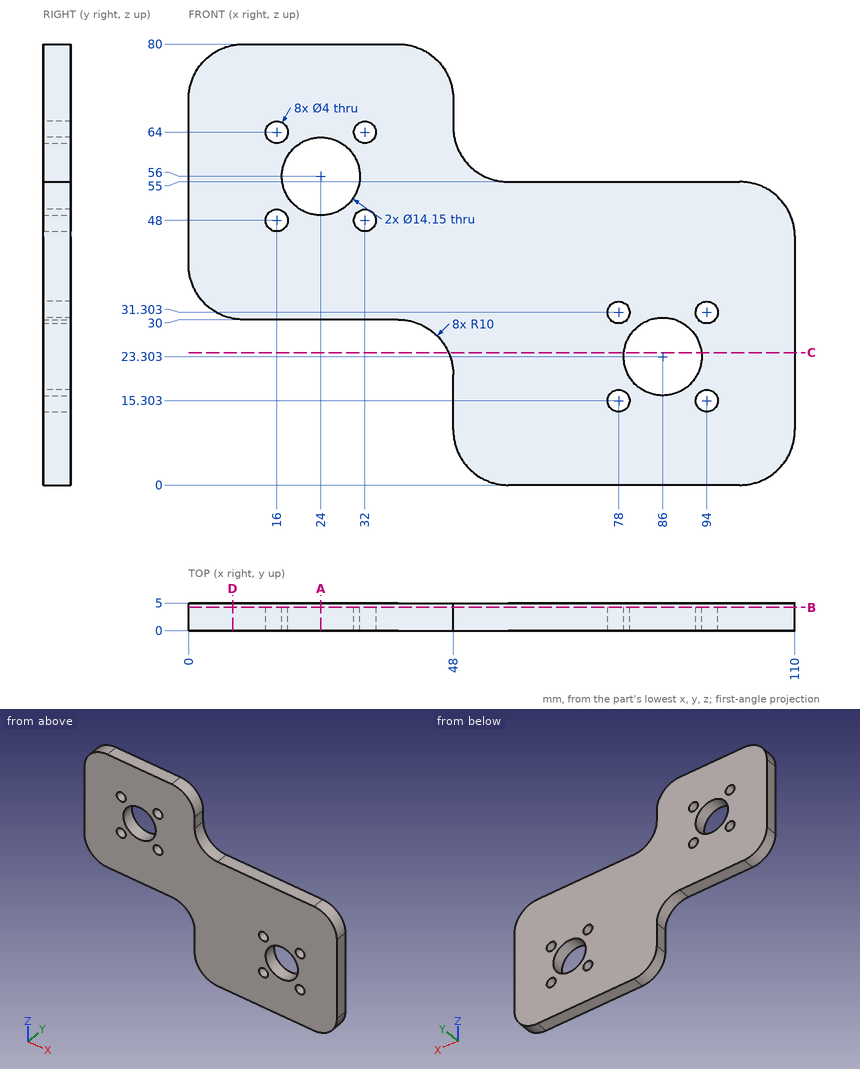
Could you check a few things on this drawing? It's one solid part, dimensions in mm from its lowest x, y, z. Give positions to 0.01 mm unless a question says otherwise; leave off trailing zeros. Loops run counter-clockwise (first coordinate to the right, second up) from the corner with the lowest first, then second, coordinate; pieces in that order, holes last. Notation, with made-up numbers: M 62.5,44.25 L 81.5,44.25 A19 ccw 81.5,59.25 Z; hole C 57,29 d4. An arc over 180 degrees is marked long. Answer as a JSON object with one key per item and string values.
Q1. Suppose I cut it at B-B, the plane y = 4.2. State how many separate pieces and enclosed holes the cut face has, plus the area to 3 significant figures.
Values found:
{"separate pieces": "1", "enclosed holes": "10", "area": "5,310 mm²"}
Q2. For P1, Ø2.5, axis at x = 19.5, y = 1.5, coming from the -Z side, with a flat end and sliding along its axis, tell me the tip position at first contact or that it passes through.
Values found:
{"P1": "stops at z = 30"}
Q3. If I drill on probe 1 along Z at (x, y) = (16, 1.7); probe 2 along X at (y, z) = (4.15, 47.5); probe 3 along X at (y, z) = (2.8, 48), over which ranges is the centre line in solid material (lowest first)? Write a range as [from, to].
Values found:
{"probe 1": "z = [30, 46], [50, 62], [66, 80]", "probe 2": "x = [0, 14.06], [17.94, 30.06], [33.94, 109.68]", "probe 3": "x = [0, 14], [18, 30], [34, 109.54]"}
Q4. Suppose I cut it at C-C, the plane z = 24. List the corners of the cut face in (x, y) for me (1 decimal), plus the area to 3 significant figures.
Values found:
{"outline": "M 47.2,0 L 79,0 L 79,5 L 47.2,5 Z; M 93,0 L 110,0 L 110,5 L 93,5 Z", "area": "244 mm²"}
Q5. Suppose I cut it at A-A, the plane x = 24. List the corners of the cut face in (y, z) for me (3 decimals).
Values found:
{"outline": "M 0,30 L 5,30 L 5,48.925 L 0,48.925 Z; M 0,63.075 L 5,63.075 L 5,80 L 0,80 Z"}
Q6. Suppose I cut it at D-D, the plane x = 8. List the corners of the cut face in (y, z) for me, plus the area to 3 significant figures.
Values found:
{"outline": "M 0,30.2 L 5,30.2 L 5,79.8 L 0,79.8 Z", "area": "248 mm²"}
